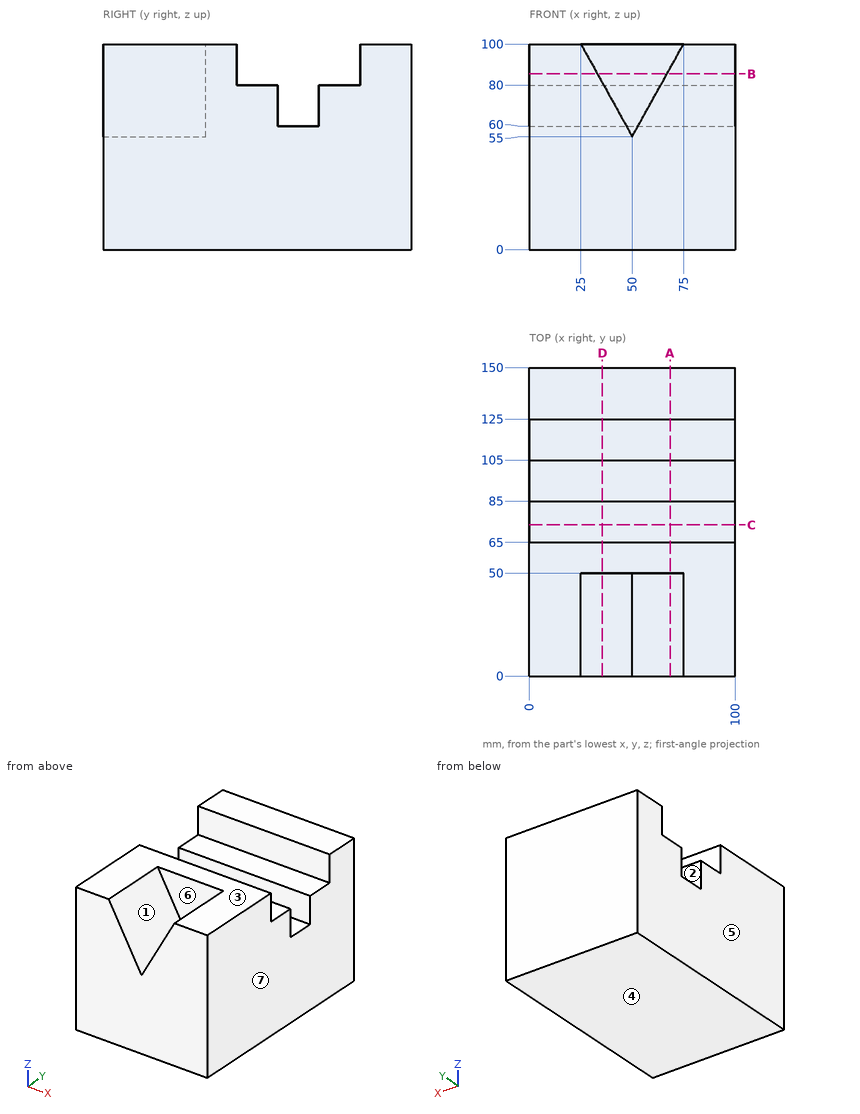
The drawing under review shows one solid part. Ordinate dimensions are in mm from its lowest x, y, z. A direction names the side the tool comes from. Round coordinates to 2 decimals unless told otherwise and drop trailing zeros. Write each loop counter-clockwise with the first axis right and the second up, starting at its lowest first coordinate (ties: lowest second). Pieces come first, ordered by that corner, then holes. Notation, with made-up numbers: (-28, -11) - (20, -11) arc R36 ccw to (20, 28) - close; hole circle Ø7 at (85.25, -15.5). An arc over 180 degrees is marked (long way). Put each result on its own line as item: value.
Q1. We need section C-C (y = 73.5). Give the boundary of the cut face in (x, z).
Solved:
outline: (0, 0) - (100, 0) - (100, 80) - (0, 80) - close
Q2. Wall thickness on probe 1 along Y at (x, z) = (71.5, 67); probe 2 along Z at (x, y) = (50.5, 113); probe 3 along X at (y, z) = (11, 68.5): over which ranges is each line inside the solid? List them lowest first.
Solved:
probe 1: y = 0 to 85, 105 to 150
probe 2: z = 0 to 80
probe 3: x = 0 to 42.5, 57.5 to 100
Q3. Machinability: for the marked faces 1, 2 and 3, which of the approach directions +Z, -Z, +X, -X, +Y, -Y give a long, thin tool a straight path to every point of the face, cutting with its end or side? Answer none if there is none.
Solved:
face 1: +Z, -Y
face 2: +Z, +X, -X
face 3: +Z, +X, -X, +Y, -Y
Q4. We need section D-D (x = 35.5). Give the boundary of the cut face in (y, z), and give its area (3 significant figures).
Solved:
outline: (0, 0) - (150, 0) - (150, 100) - (125, 100) - (125, 80) - (105, 80) - (105, 60) - (85, 60) - (85, 80) - (65, 80) - (65, 100) - (50, 100) - (50, 81.1) - (0, 81.1) - close
area: 12,500 mm2
Q5. Mouldability with a two-part tool opening along X and no side actions: class the marked faces 4, 5, 6 and 7 as released by +X, released by -X, zero draft, split by the parting line, or undercut.
Solved:
face 4: zero draft
face 5: released by -X
face 6: undercut
face 7: released by +X
Q6. We need section B-B (z = 85.5). Give the boundary of the cut face in (x, y), and give its area (3 significant figures).
Solved:
outline: (0, 0) - (33.06, 0) - (33.06, 50) - (66.94, 50) - (66.94, 0) - (100, 0) - (100, 65) - (0, 65) - close; (0, 125) - (100, 125) - (100, 150) - (0, 150) - close
area: 7,310 mm2
Q7. We need section A-A (x = 68.5). Give the boundary of the cut face in (y, z).
Solved:
outline: (0, 0) - (150, 0) - (150, 100) - (125, 100) - (125, 80) - (105, 80) - (105, 60) - (85, 60) - (85, 80) - (65, 80) - (65, 100) - (50, 100) - (50, 88.3) - (0, 88.3) - close
Q8. Insertion check: pin 1 Ø6 at (x, y) = (61, 92.5) entering from +Z; pin 2 Ø6 at (x, y) = (58.5, 75.5) entering from +Z. Each pin has a flat end and moves straight along its axis. Give the tip position at first contact, or say it passes through.
Solved:
pin 1: stops at z = 60
pin 2: stops at z = 80
